Geometry: final body of the model. Coordinates: model frame, mm. A direction names the side the tool comes from. Give positions to 0.01 mm unless a question says otherwise; leave off trailing zeros. Order: outer loops, then holes, each group sorted by start corner. A loop starts at its lowest first (then second) coordinate and runs counter-clockwise, first axis right, second up. Notation, with made-up numbers: (57, -27.5) - (85, -27.5) arc R15 cw to (85, -10.5) - close; hole circle Ø4 at (81, 23). An arc over 180 degrees is marked (long way). Put each result on its own line as item: value. Start each with the question number.
1. Section A-A on x = 0. Return the cut outline in (y, z) (3 decimals).
2. Section C-C on z = 14.5. Return the cut outline in (x, y) (3 decimals).
3. Mould query, pull axis Y, two halves, no side actions, for faces 1 (the flat face through (3.175, 14, 16)), 2 (the cylindrical face through (-4.8, -21.7, 15.7)), 3 (the flat face through (10, -10, 31.75)). Classes: pulls with the +Y half, pulls with the -Y half, needs draft (parallel to the pull), parting line crosses it, or undercut.
4. Section D-D on y = 14. Return the cut outline in (x, z) (3 decimals).
5. Set-up query: faces 4 (the flat face through (-15.875, 27, 6)), 5 (the flat face through (15.875, 27, 6)), 6 (the flat face through (-0.3, 16.4, 0)), 7 (the cylindrical face through (0.35, 53.97, 6.26)), 8 (the flat face through (0, 15.875, 16)). Return all of +Z, -Z, +X, -X, +Y, -Y with unobstructed straight access to the full face (end or side cutting, diameter ignored); none if empty.
6. First-contact query: P1, Ø5, axis at x = 1, z = 13.5, coming from the -Y side (3 decimals); P2, Ø6.5, axis at y = 25, z = 3.5, coming from the -X side (3 decimals); P3, Ø5, axis at y = -5, z = 16.5, coming from the +X side. Flat tips, straight axial feed; report the tip coordinate or a pass-through.
7. Section B-B on y = 0. Return the cut outline in (x, z) (3 decimals).
8. Ray query, line 1 along Y through (x, z) = (0, 12) (3 decimals); line 2 along Y through (x, z) = (3, 8.5) (3 decimals); line 3 along X through (y, z) = (0, 25.5) (3 decimals). Return the intervals inside material, ascending. Write a range as from..to.
from build123d import *

# Parameters (mm, degrees)
SKETCH1_R           = 22.225
BOSS_EXTRUDE1_DEPTH = 31.75
SKETCH2_R           = 6.35
BOSS_EXTRUDE2_DEPTH = 12.7
CUT_EXTRUDE1_DEPTH  = 67.447827278


with BuildPart() as part:
    # Sketch1 → Boss-Extrude1 (new body)
    with BuildSketch(Plane.XY):
        Circle(SKETCH1_R)
    extrude(amount=BOSS_EXTRUDE1_DEPTH)

    # Sketch2 → Boss-Extrude2 (add)
    with BuildSketch(Plane.XY):
        with BuildLine():
            Line((-15.875, 7.271721018), (15.875, 7.271721018))
            Line((15.875, 7.271721018), (15.875, 38.1))
            ThreePointArc((15.875, 38.1), (0, 53.975), (-15.875, 38.1))
            Line((-15.875, 38.1), (-15.875, 7.271721018))
        make_face()
        with Locations((0, 38.1)):
            Circle(SKETCH2_R, mode=Mode.SUBTRACT)
    extrude(amount=BOSS_EXTRUDE2_DEPTH)

    # Sketch3 → Cut-Extrude1 (cut, through all)
    with BuildSketch(Plane.XY.offset(31.75)):
        with BuildLine():
            Line((-3.175, 12.564048608), (-3.175, 15.875))
            Line((-3.175, 15.875), (3.175, 15.875))
            Line((3.175, 15.875), (3.175, 12.564048608))
            ThreePointArc((3.175, 12.564048608), (0, -12.959010086), (-3.175, 12.564048608))
        make_face()
    extrude(amount=-CUT_EXTRUDE1_DEPTH, mode=Mode.SUBTRACT)


solid = part.part
Resolved:
1. outline: (-22.225, 0) - (-12.959, 0) - (-12.959, 31.75) - (-22.225, 31.75) - close; (15.875, 0) - (31.75, 0) - (31.75, 12.7) - (22.225, 12.7) - (22.225, 31.75) - (15.875, 31.75) - close; (44.45, 0) - (53.975, 0) - (53.975, 12.7) - (44.45, 12.7) - close
2. outline: circle Ø44.45 at (0, 0); hole (-3.175, 12.564) arc R12.959 ccw (long way) to (3.175, 12.564) - (3.175, 15.875) - (-3.175, 15.875) - close
3. face 1: undercut
3. face 2: parting line crosses it
3. face 3: needs draft
4. outline: (-17.261, 0) - (-3.175, 0) - (-3.175, 31.75) - (-17.261, 31.75) - close; (3.175, 0) - (17.261, 0) - (17.261, 31.75) - (3.175, 31.75) - close
5. face 4: +Z, -Z, -X, +Y
5. face 5: +Z, -Z, +X, +Y
5. face 6: -Z, +X, -X, +Y, -Y
5. face 7: +Z, -Z, +Y
5. face 8: +Z, -Z
6. P1: y = -22.225
6. P2: x = -15.875
6. P3: x = 22.08
7. outline: (-22.225, 0) - (-12.959, 0) - (-12.959, 31.75) - (-22.225, 31.75) - close; (12.959, 0) - (22.225, 0) - (22.225, 31.75) - (12.959, 31.75) - close
8. line 1: -22.225..-12.959, 15.875..31.75, 44.45..53.975
8. line 2: -22.022..-12.607, 15.875..32.503, 43.697..53.689
8. line 3: -22.225..-12.959, 12.959..22.225
